```python
from build123d import *

# Parameters (mm, degrees)
SKETCH1_R                   = 12
BOSS_EXTRUDE1_DEPTH         = 3
TAP_DRILL_FOR_M3_TAP1_D     = 2.5
TAP_DRILL_FOR_M3_TAP1_DEPTH = 5
TAP_DRILL_FOR_M3_TAP1_TIP   = 0.751075774
TAP_DRILL_FOR_M4_TAP1_D     = 3.3
TAP_DRILL_FOR_M4_TAP1_DEPTH = 5
TAP_DRILL_FOR_M4_TAP1_TIP   = 0.991420021
FILLET1_R                   = 2
TAP_DRILL_FOR_M2_TAP1_D     = 1.6
TAP_DRILL_FOR_M2_TAP1_DEPTH = 5
TAP_DRILL_FOR_M2_TAP1_TIP   = 0.480688495
CUT_EXTRUDE1_DEPTH          = 10


with BuildPart() as part:
    # Sketch1 → Boss-Extrude1 (new body)
    with BuildSketch(Plane.XY):
        Polygon((18.05, -56.055), (18.05, -21.05), (21.05, -18.05), (21.05, 18.05), (18.05, 21.05), (-18.05, 21.05), (-21.05, 18.05), (-21.05, -18.05), (-18.05, -21.05), (-18.05, -56.055), align=None)
        Circle(SKETCH1_R, mode=Mode.SUBTRACT)
    extrude(amount=BOSS_EXTRUDE1_DEPTH)

    # Tap Drill for M3 Tap1
    with Locations(Plane.XY.offset(3)):
        with Locations((-15.5, 15.5), (15.5, 15.5), (-15.5, -15.5), (15.5, -15.5)):
            Hole(TAP_DRILL_FOR_M3_TAP1_D / 2, depth=TAP_DRILL_FOR_M3_TAP1_DEPTH)
            with Locations((0, 0, -(TAP_DRILL_FOR_M3_TAP1_DEPTH + TAP_DRILL_FOR_M3_TAP1_TIP / 2))):  # 118° drill point
                Cone(0, TAP_DRILL_FOR_M3_TAP1_D / 2, TAP_DRILL_FOR_M3_TAP1_TIP, mode=Mode.SUBTRACT)

    # Tap Drill for M4 Tap1
    with Locations(Plane.XY.offset(3)):
        with Locations((12, -41.055), (-12, -41.055)):
            Hole(TAP_DRILL_FOR_M4_TAP1_D / 2, depth=TAP_DRILL_FOR_M4_TAP1_DEPTH)
            with Locations((0, 0, -(TAP_DRILL_FOR_M4_TAP1_DEPTH + TAP_DRILL_FOR_M4_TAP1_TIP / 2))):  # 118° drill point
                Cone(0, TAP_DRILL_FOR_M4_TAP1_D / 2, TAP_DRILL_FOR_M4_TAP1_TIP, mode=Mode.SUBTRACT)

    # Fillet1
    fillet1_edges = [part.edges().sort_by_distance(p)[0] for p in [
        (18.05, -21.05, 1.5),
        (18.05, -56.055, 1.5),
        (-18.05, -56.055, 1.5),
        (-18.05, -21.05, 1.5),
    ]]
    fillet(fillet1_edges, radius=FILLET1_R)

    # Tap Drill for M2 Tap1
    with Locations(Plane.XY.offset(3)):
        with Locations((10.52945603, -21.86131015), (10.52945603, -28.56131015)):
            Hole(TAP_DRILL_FOR_M2_TAP1_D / 2, depth=TAP_DRILL_FOR_M2_TAP1_DEPTH)
            with Locations((0, 0, -(TAP_DRILL_FOR_M2_TAP1_DEPTH + TAP_DRILL_FOR_M2_TAP1_TIP / 2))):  # 118° drill point
                Cone(0, TAP_DRILL_FOR_M2_TAP1_D / 2, TAP_DRILL_FOR_M2_TAP1_TIP, mode=Mode.SUBTRACT)

    # Sketch8 → Cut-Extrude1 (cut)
    with BuildSketch(Plane.XY):
        with BuildLine():
            Line((-0.350833888, -40.786266358), (3.496510612, -35.314487513))
            ThreePointArc((3.496510612, -35.314487513), (3.110982416, -33.102773131), (0.899268034, -33.488301326))
            Line((0.899268034, -33.488301326), (0.384994593, -34.219712442))
            Line((0.384994593, -34.219712442), (-0.509366672, -33.296697877))
            ThreePointArc((-0.509366672, -33.296697877), (-2.754151719, -33.261305914), (-2.789543683, -35.506090962))
            Line((-2.789543683, -35.506090962), (-1.474067559, -36.863711947))
            Line((-1.474067559, -36.863711947), (-2.948076466, -38.96008017))
            ThreePointArc((-2.948076466, -38.96008017), (-2.562548271, -41.171794553), (-0.350833888, -40.786266358))
        make_face()
    extrude(amount=CUT_EXTRUDE1_DEPTH, mode=Mode.SUBTRACT)


solid = part.part
```
The model under review builds one solid part; all positions refer to its coordinate system, in mm. A direction names the side the tool comes from. Round coordinates to 2 decimals unless told otherwise and drop trailing zeros. Loops run counter-clockwise (first coordinate to the right, second up) from the corner with the lowest first, then second, coordinate; pieces in that order, holes last. Notation, with made-up numbers: M 56,68 L 70,68 A19 ccw 70,103 Z; hole C 2,29 d9. An arc over 180 degrees is marked long. Answer as a JSON object with one key per item and string values.
(1) Take a section at A-A on y = 15.5. Give the boundary of the cut face in (x, z).
Resolved:
{"outline": "M -21.05,0 L -16.75,0 L -16.75,3 L -21.05,3 Z; M -14.25,0 L 14.25,0 L 14.25,3 L -14.25,3 Z; M 16.75,0 L 21.05,0 L 21.05,3 L 16.75,3 Z"}
(2) Tool access review of faces 1 (the flat face through (-2.201, -37.897, 1.479)), 2 (the flat face through (18.05, -38, 1)), 3 (the flat face through (0, -17, 0)): name each direction out of +Z, -Z, +X, -X, +Y, -Y from which nothing blocks a thin tool from reaching the whole face with its end or side.
Resolved:
{"face 1": "+Z, -Z", "face 2": "+Z, -Z, +X, -Y", "face 3": "-Z, +X, -X, +Y, -Y"}
(3) Take a section at B-B on y = 0. Give the boundary of the cut face in (x, z).
Resolved:
{"outline": "M -21.05,0 L -12,0 L -12,3 L -21.05,3 Z; M 12,0 L 21.05,0 L 21.05,3 L 12,3 Z"}
(4) Take a section at C-C on x = 5.5. Give the boundary of the cut face in (y, z) (3 decimals).
Resolved:
{"outline": "M -56.055,0 L -10.665,0 L -10.665,3 L -56.055,3 Z; M 10.665,0 L 21.05,0 L 21.05,3 L 10.665,3 Z"}
(5) To check wall thickness, follow line 1 along Y through (x, z) = (-15.5, 1.1) (3 decimals); line 2 along Y through (x, z) = (2, 0.45) (3 decimals); line 3 along Y through (x, z) = (10, 1.6) (3 decimals). State the ranges of each line that lie inside material, in increasing order.
Resolved:
{"line 1": "-56.055 to -16.75, -14.25 to 14.25, 16.75 to 21.05", "line 2": "-56.055 to -37.443, -32.826 to -11.832, 11.832 to 21.05", "line 3": "-56.055 to -29.161, -27.962 to -22.461, -21.262 to -6.633, 6.633 to 21.05"}
(6) Draft analysis for pull direction X (two halves, no side actions). For faces 4 (the cylindrical face through (18.2, -21.12, 1.52)), 5 (the flat face through (-2.141, -36.175, 1.479)), 6 (the flat face through (0, -56.055, 1)), 7 (the flat face through (1.546, -38.089, 1.479)), state which applies: released by +X, released by -X, zero draft, split by the parting line, or undercut.
Resolved:
{"face 4": "released by +X", "face 5": "undercut", "face 6": "zero draft", "face 7": "undercut"}
(7) Take a section at D-D on z = 2.35. Count the separate pieces of the cut face and the enclosed holes in it, and give its area (3 significant figures).
Resolved:
{"separate pieces": "1", "enclosed holes": "10", "area": "2,490 mm²"}
